Autodesk Inventor part; units mm, degrees
ref_plane "YZ Plane" through (0, 0, 0) normal (1, 0, 0) x (0, 1, 0)
ref_plane "XZ Plane" through (0, 0, 0) normal (0, 1, 0) x (-1, 0, 0)
ref_plane "XY Plane" through (0, 0, 0) normal (0, 0, 1) x (1, 0, 0)
sketch "Sketch1" plane through (0, 0, 0) normal (0, 1, 0) x (-1, 0, 0)
  circle A0 centre (0, 0) radius 6.35 construction
  line L0 (6.35, -3.6662) -> (0, -7.3323)
  line L1 (0, -7.3323) -> (-6.35, -3.6662)
  line L2 (-6.35, -3.6662) -> (-6.35, 3.6662)
  line L3 (-6.35, 3.6662) -> (0, 7.3323)
  line L4 (0, 7.3323) -> (6.35, 3.6662)
  line L5 (6.35, 3.6662) -> (6.35, -3.6662)
  circle A1 centre (0, 0) radius 9.525
  point P0 (6.35, 0)
  dimension "d0" = 12.7
  dimension "d1" = 19.05
extrude "Extrusion1" add sketch "Sketch1" along normal blind 31.75
properties part number "SportGearbox_HexDiffGearSpacer"
For this review, take the finished solid that the model builds, in its own axes (mm). A direction names the side the tool comes from. Round coordinates to 2 decimals unless told otherwise and drop trailing zeros. Write each loop counter-clockwise with the first axis right and the second up, starting at its lowest first coordinate (ties: lowest second). Pieces come first, ordered by that corner, then holes. Notation, with made-up numbers: (76.5, 64) -> (109.5, 64) arc R5 ccw to (109.5, 69) -> close; hole circle Ø10 at (19, -17). An arc over 180 degrees is marked (long way). One line per question, with ' | ' between items. Start each with the question number.
1) Mouldability with a two-part tool opening along Z and no side actions: class faces 3 (the cylindrical face through (7.559, 15.653, 5.796)), 4 (the flat face through (2.3, 31.75, -6.2)), 5 (the flat face through (3.219, 15.653, 5.474)) as +Z half, -Z half, draft (parallel to the pull), parting line (faces both ways), or undercut.
2) Machinability: for faces 1 (the flat face through (2.3, 0, -6.2)), 2 (the flat face through (6.35, 16, 0)), which of the approach directions +Z, -Z, +X, -X, +Y, -Y give a long, thin tool a straight path to every point of the face, cutting with its end or side? Answer none if there is none.
3) Add section B-B (x = -1.5). Write out the cut boundary in (y, z).
4) Add section C-C (y = 24). Write out the cut boundary in (x, z) (3 decimals), and give its area (3 significant figures).
5) For pin 1 Ø2 at (y, z) = (4, -2.5) entering from +X; pin 2 Ø10 at (x, y) = (-5.5, 25) entering from +Z; pin 3 Ø1 at (y, z) = (17.5, 1.5) entering from -X, all flat-tipped, find the tip position at first contact; note any pin that passes through.
6) Add section D-D (x = 7.5). Write out the cut boundary in (y, z), and give its area (3 significant figures).
7) Add section A-A (z = 0). Write out the cut boundary in (x, y) (3 decimals).
8) Wall thickness on line 1 along X through (y, z) = (11, 3.25); line 2 along Z through (x, y) = (-2.75, 24.5); line 3 along Z through (x, y) = (-4.5, 23): over which ranges is each line inside the solid? List them lowest first.
Reported:
1) face 3: parting line | face 4: draft | face 5: undercut
2) face 1: +Z, -Z, +X, -X, -Y | face 2: +Y, -Y
3) outline: (0, -9.41) -> (31.75, -9.41) -> (31.75, -6.47) -> (0, -6.47) -> close; (0, 6.47) -> (31.75, 6.47) -> (31.75, 9.41) -> (0, 9.41) -> close
4) outline: circle Ø19.05 at (0, 0); hole (-6.35, -3.666) -> (0, -7.332) -> (6.35, -3.666) -> (6.35, 3.666) -> (0, 7.332) -> (-6.35, 3.666) -> close | area: 145 mm²
5) pin 1: stops at x = 9.41 | pin 2: stops at z = 9.51 | pin 3: stops at x = -9.47
6) outline: (0, -5.87) -> (31.75, -5.87) -> (31.75, 5.87) -> (0, 5.87) -> close | area: 373 mm²
7) outline: (-9.525, 0) -> (-6.35, 0) -> (-6.35, 31.75) -> (-9.525, 31.75) -> close; (6.35, 0) -> (9.525, 0) -> (9.525, 31.75) -> (6.35, 31.75) -> close
8) line 1: x = -8.95 to -6.35, 6.35 to 8.95 | line 2: z = -9.12 to -5.74, 5.74 to 9.12 | line 3: z = -8.39 to -4.73, 4.73 to 8.39
